```python
from build123d import *

# Parameters (mm, degrees)
SKETCH1_R           = 3.2639
BOSS_EXTRUDE1_DEPTH = 6.35
FILLET1_R           = 6.35
SKETCH2_R           = 3.2639
CUT_EXTRUDE2_DEPTH  = 375.272921719
SKETCH3_R           = 3.2639
CUT_EXTRUDE3_DEPTH  = 375.272921719
FILLET2_R           = 6.35


with BuildPart() as part:
    # Sketch1 → Boss-Extrude1 (new, symmetric)
    with BuildSketch(Plane.XY):
        with BuildLine():
            Line((-323.85, -18.447144741), (-171.45, -18.447144741))
            ThreePointArc((-171.45, -18.447144741), (0, 52.569770528), (171.45, -18.447144741))
            Line((171.45, -18.447144741), (323.85, -18.447144741))
            Line((323.85, -18.447144741), (323.85, 32.352855259))
            Line((323.85, 32.352855259), (349.25, 32.352855259))
            Line((349.25, 32.352855259), (349.25, 57.752855259))
            Line((349.25, 57.752855259), (300.0375, 57.752855259))
            Line((300.0375, 57.752855259), (300.0375, 51.402855259))
            Line((300.0375, 51.402855259), (171.45, 51.402855259))
            Line((171.45, 51.402855259), (171.45, 57.752855259))
            Line((171.45, 57.752855259), (152.4, 133.952855259))
            Line((152.4, 133.952855259), (88.9, 133.952855259))
            Line((88.9, 133.952855259), (88.9, 95.776655259))
            Line((88.9, 95.776655259), (76.2, 95.776655259))
            Line((76.2, 95.776655259), (76.2, 133.952855259))
            Line((76.2, 133.952855259), (-76.2, 133.952855259))
            Line((-76.2, 133.952855259), (-76.2, 95.776655259))
            Line((-76.2, 95.776655259), (-88.9, 95.776655259))
            Line((-88.9, 95.776655259), (-88.9, 133.952855259))
            Line((-88.9, 133.952855259), (-152.4, 133.952855259))
            Line((-152.4, 133.952855259), (-171.45, 57.752855259))
            Line((-171.45, 57.752855259), (-171.45, 51.402855259))
            Line((-171.45, 51.402855259), (-300.0375, 51.402855259))
            Line((-300.0375, 51.402855259), (-300.0375, 57.752855259))
            Line((-300.0375, 57.752855259), (-349.25, 57.752855259))
            Line((-349.25, 57.752855259), (-349.25, 32.352855259))
            Line((-349.25, 32.352855259), (-323.85, 32.352855259))
            Line((-323.85, 32.352855259), (-323.85, -18.447144741))
        make_face()
        with Locations((-336.55, 45.052855259)):
            Circle(SKETCH1_R, mode=Mode.SUBTRACT)
        with Locations(Location((336.55, 45.052855259, 0), (0, 0, 180))):
            Circle(SKETCH1_R, mode=Mode.SUBTRACT)
    extrude(amount=BOSS_EXTRUDE1_DEPTH, both=True)

    # Fillet1
    fillet1_edges = [part.edges().sort_by_distance(p)[0] for p in [
        (88.9, 95.776655259, 0),
        (76.2, 95.776655259, 0),
        (-88.9, 95.776655259, 0),
        (-76.2, 95.776655259, 0),
        (323.85, 32.352855259, 0),
        (171.45, 51.402855259, 0),
        (300.0375, 51.402855259, 0),
        (-171.45, 51.402855259, 0),
        (-300.0375, 51.402855259, 0),
        (-323.85, 32.352855259, 0),
    ]]
    fillet(fillet1_edges, radius=FILLET1_R - 0.0001)  # a hair under: the kernel refuses the full size

    # Sketch2 → Cut-Extrude2 (cut, through all)
    with BuildSketch(Plane.XY.offset(6.35)):
        with Locations((-234.95, 17.366855259)):
            Circle(SKETCH2_R)
        with Locations((-234.95, 34.384855259)):
            Circle(SKETCH2_R)
        with Locations((234.95, 34.384855259)):
            Circle(SKETCH2_R)
        with Locations((234.95, 17.366855259)):
            Circle(SKETCH2_R)
    extrude(amount=-CUT_EXTRUDE2_DEPTH, mode=Mode.SUBTRACT)

    # Sketch3 → Cut-Extrude3 (cut, through all)
    with BuildSketch(Plane.XY.offset(6.35)):
        with Locations((-101.6, 64.198647102)):
            Circle(SKETCH3_R)
        with Locations((101.6, 64.198647102)):
            Circle(SKETCH3_R)
        with Locations((-62.834515607, 64.198647102)):
            Circle(SKETCH3_R)
        with Locations(Location((62.834515607, 64.198647102, 0), (0, 0, 180))):
            Circle(SKETCH3_R)
    extrude(amount=-CUT_EXTRUDE3_DEPTH, mode=Mode.SUBTRACT)

    # Fillet2
    fillet2_edges = [part.edges().sort_by_distance(p)[0] for p in [
        (-152.4, 133.952855259, 0),
        (-88.9, 133.952855259, 0),
        (-76.2, 133.952855259, 0),
        (76.2, 133.952855259, 0),
        (88.9, 133.952855259, 0),
        (152.4, 133.952855259, 0),
        (300.0375, 57.752855259, 0),
        (349.25, 57.752855259, 0),
        (349.25, 32.352855259, 0),
        (323.85, -18.447144741, 0),
        (171.45, -18.447144741, 0),
        (-171.45, -18.447144741, 0),
        (-323.85, -18.447144741, 0),
        (-349.25, 32.352855259, 0),
        (-349.25, 57.752855259, 0),
        (-300.0375, 57.752855259, 0),
    ]]
    fillet(fillet2_edges, radius=FILLET2_R)


solid = part.part
```
The listing builds one solid part. Answer for the finished solid, in the listing's coordinates (mm). A direction names the side the tool comes from. Give positions to 0.01 mm unless a question says otherwise; leave off trailing zeros. Write each loop counter-clockwise with the first axis right and the second up, starting at its lowest first coordinate (ties: lowest second). Pieces come first, ordered by that corner, then holes. Notation, with made-up numbers: M 84.5,-34.75 L 129.5,-34.75 A26 cw 129.5,-2.75 Z; hole C 60.25,65 d6. An arc over 180 degrees is marked long. Write each question's results on one line, items separated by ' | '.
Q1. Consider L1, parallel to Y at x = -234.95, z = -2.5; L2, parallel to X at y = 126, z = -4.25; L3, parallel to Y at x = -101.6, z = 2.25. Determine where each line is inside the solid, lowest interval first. Write a range as from..to.
Output values:
L1: -18.45..14.1, 20.63..31.12, 37.65..51.4 | L2: -154.39..-88.9, -76.2..76.2, 88.9..154.39 | L3: 30.26..60.93, 67.46..133.95
Q2. Section D-D, the plane y = 77 is taken. Write down the section's boundary in (x, z), then the cut area to 3 significant figures.
Output values:
outline: M -166.64,-6.35 L 166.64,-6.35 L 166.64,6.35 L -166.64,6.35 Z | area: 4,230 mm2
Q3. Section B-B, the plane x = -278 is taken. Write down the section's boundary in (y, z).
Output values:
outline: M -18.45,-6.35 L 51.4,-6.35 L 51.4,6.35 L -18.45,6.35 Z
Q4. Section A-A, the plane y = 111 is taken. Write down the section's boundary in (x, z).
Output values:
outline: M -158.14,-6.35 L -88.9,-6.35 L -88.9,6.35 L -158.14,6.35 Z; M -76.2,-6.35 L 76.2,-6.35 L 76.2,6.35 L -76.2,6.35 Z; M 88.9,-6.35 L 158.14,-6.35 L 158.14,6.35 L 88.9,6.35 Z
Q5. Section C-C, the plane z = -4 is taken. Count the separate pieces of the cut face and the enclosed holes in it, then the cut area to 3 significant figures.
Output values:
separate pieces: 1 | enclosed holes: 10 | area: 55,600 mm2
Q6. Flat-ended cylindrical pins translate along their axes: P1, Ø4, axis at x = -62.83, y = 64.2, coming from the +Z side; P2, Ø1, axis at x = 20, z = -1, coming from the -Y side; P3, Ø4, axis at x = 335, z = 1.5, coming from the -Y side; P4, Ø4, axis at y = 112, z = 1.5, coming from the +X side. Find the tip coordinate at first contact, or state that the pin passes through.
Output values:
P1: through | P2: y = 51.7 | P3: y = 32.35 | P4: x = 158.39
Q7. A tool of negligible diameter and unlimited length cuts with its end or side. For faces 1 (the flat face through (336, 32.353, 0)), 2 (the flat face through (237, 51.403, 0)), 3 (the flat face through (-324, 57.753, 0)), 4 (the flat face through (-337, 32.353, 0)), from which of +Z, -Z, +X, -X, +Y, -Y can it reach the whole face along a straight path? Write none if from no direction.
Output values:
face 1: +Z, -Z, +X, -Y | face 2: +Z, -Z, +Y | face 3: +Z, -Z, -X, +Y | face 4: +Z, -Z, -X, -Y
